Verification items for the finished model (mm, model axes). Face numbers are marked on the shaded views. A direction names the side the tool comes from. Coordinates: 2 decimals unless noted, no trailing zeros. Order: outer loops, then holes, each group sorted by start corner. A loop starts at its lowest first (then second) coordinate and runs counter-clockwise, first axis right, second up. Notation, with made-up numbers: M 78,56 L 104,56 A16 cw 104,63 Z; hole C -11.75,70 d3. An arc over 180 degrees is marked long. Return JSON: item names as keys, results as strings. Group by question number.
Q1. Thickness scan on probe 1 along Y at (x, z) = (-2, 33); probe 2 along Z at (x, y) = (-7.5, 17.5); probe 3 along X at (y, z) = (1, 36.83) (3 decimals). Record the ranges inside material, lowest first.
Q2. Section check B-B, the plane x = 1.25. Enter the section's corners in (y, z).
Q3. Section check A-A, the plane x = 5. Enter the section's corners in (y, z), then the cut area to 3 significant figures.
Q4. Access from +Z, -Z, +X, -X, +Y, -Y to the whole of each face (thin tool, end or side, straight path). Record for the marked faces 1, 2 and 3.
Q5. Section check C-C, the plane z = 36.83. Enter the section's corners in (x, y) (3 decimals).
Q6. Mould release check, pull along Y, two halves, no side actions. Record for the marked faces 4, 5 and 6: pulls with the +Y half, pulls with the -Y half, needs draft (parallel to the pull), parting line crosses it, or undercut.
Q7. Go/stop test with flat-tipped pins: pin 1 Ø1.1 at (x, z) = (6.985, 36.83) entering from +Y; pin 2 Ø2.5 at (y, z) = (-7, 31) entering from -X (3 decimals); pin 3 Ø3 at (y, z) = (-15.5, 29) entering from -X (3 decimals). Record where each tip stops, or that it passes through.
from build123d import *

# Parameters (mm, degrees)
F0_W        = 19.05
F0_H        = 50.8
F1_DEPTH    = 38.1
F2_R        = 5.08
F3_W        = 5.08
F3_H        = 20.32
F4_DEPTH    = 50.8
F5_T        = 2.54
F5_T3_DEPTH = 55.88
F6_R        = 5.07999
F7_R        = 0.635
F8_DEPTH    = 21.59


# Not quite as in the source:
# - a fillet or chamfer is up to 0.001 mm smaller than in the source, because OpenCascade refuses the exact size
# - a shell that OpenCascade refuses in one call is made with other operations: the cavity is built on its own and cut out


with BuildPart() as f1:
    # F0 (on Top) → F1 (new body)
    with BuildSketch(Plane.XY):
        Rectangle(F0_W, F0_H)
    extrude(amount=F1_DEPTH)

    # F2
    f2_edges = [f1.edges().sort_by_distance(p)[0] for p in [
        (0, -25.4, 38.1),
        (0, 25.4, 38.1),
        (-9.525, -25.4, 19.05),
        (-9.525, 0, 38.1),
        (-9.525, 25.4, 19.05),
    ]]
    fillet(f2_edges, radius=F2_R)

    # F3 (on face) → F4 (cut)
    with BuildSketch(Plane.XZ.offset(25.4)):
        with Locations((6.985, 15.24)):
            Rectangle(F3_W, F3_H)
    extrude(amount=-F4_DEPTH, mode=Mode.SUBTRACT)

    # F5: shell of thickness 2.54, made by hand


with BuildPart() as f5_core1:
    # F5_t2: copy of F1
    add(f1.part)

    # the walls: a layer under each face that stays
    f5_faces = [f5_core1.faces().sort_by_distance(p)[0] for p in [
        (2.54, -25.4, 16.51),
        (9.525, 0, 2.54),
        (6.985, 0, 5.08),
        (4.445, 0, 15.24),
        (6.985, 0, 25.4),
        (9.525, 0, 31.75),
        (2.54, -23.9121024484, 36.6121024484),
        (-8.0371024484, -23.9121024484, 16.51),
        (0, 0, 0),
        (2.54, 25.4, 16.51),
        (2.54, 23.9121024484, 36.6121024484),
        (-8.0371024484, -22.86, 35.56),
        (-8.0371024484, 23.9121024484, 16.51),
        (-8.0371024484, 22.86, 35.56),
    ]]
    thicken(f5_faces, amount=-F5_T, mode=Mode.SUBTRACT)

    # F5_s4 → F5_t3 (cut)
    with BuildSketch(Plane.XZ.offset(-27.94)):
        Polygon((4.4704, 5.1054), (4.445, 2.54), (1.905, 2.54), (1.905, 5.08), align=None)
        Polygon((4.4704, 25.3746), (1.905, 25.4), (1.905, 27.94), (4.445, 27.94), align=None)
    extrude(amount=F5_T3_DEPTH, mode=Mode.SUBTRACT)


with BuildPart() as f1_1:
    add(f1.part)

    # what is left inside the walls is the cavity
    f5_cavity = [f5_core1.part.solids().sort_by_distance(p)[0] for p in [
        (-9.4996, 0, 22.86),
    ]]
    add(f5_cavity, mode=Mode.SUBTRACT)

    # F6 (radius 5.08 in the source; OpenCascade refuses exactly that, so slightly less here)
    f6_edges = [f1_1.edges().sort_by_distance(p)[0] for p in [
        (4.445, 0, 5.08),
        (4.445, 0, 25.4),
    ]]
    fillet(f6_edges, radius=F6_R)

    # F7 (on Front) → F8 (cut, symmetric)
    with BuildSketch(Plane.XZ):
        with Locations((6.985, 36.83)):
            Circle(F7_R)
    extrude(amount=F8_DEPTH, both=True, mode=Mode.SUBTRACT)


solid = f1_1.part
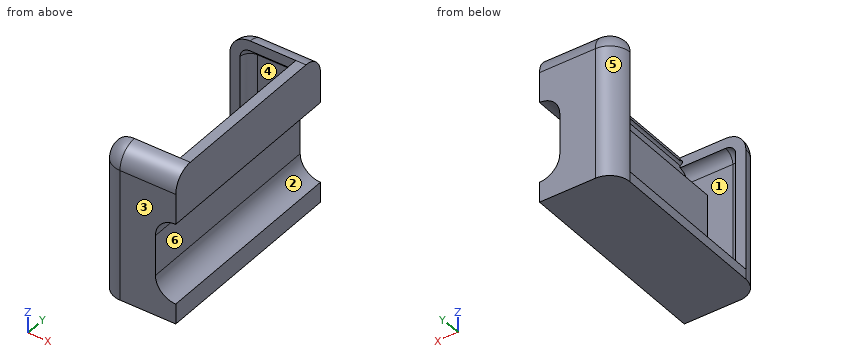
Numbers:
{
 "1": {"probe 1": "y = -25.4 to -22.86, 22.86 to 25.4", "probe 2": "z = 0 to 2.54", "probe 3": "x = 7.62 to 9.525"},
 "2": {"outline": "M -25.4,0 L 25.4,0 L 25.4,33.02 A5.08 ccw 20.32,38.1 L 20.32,35.56 A2.54 cw 22.86,33.02 L 22.86,2.54 L -22.86,2.54 L -22.86,33.02 A2.54 cw -20.32,35.56 L -20.32,38.1 A5.08 ccw -25.4,33.02 Z"},
 "3": {"outline": "M -25.4,0 L 25.4,0 L 25.4,7.85 L -25.4,7.85 Z; M -25.4,22.63 L 25.4,22.63 L 25.4,33.02 A5.08 ccw 20.32,38.1 L 20.32,35.56 A2.54 cw 22.86,33.02 L 22.86,27.94 L -22.86,27.94 L -22.86,33.02 A2.54 cw -20.32,35.56 L -20.32,38.1 A5.08 ccw -25.4,33.02 Z", "area": "725 mm2"},
 "4": {"face 1": "none", "face 2": "+X, +Y, -Y", "face 3": "+Z, -Z, +X, -X, -Y"},
 "5": {"outline": "M -7.805,-20.32 A3.36 ccw -4.445,-23.68 L 9.525,-23.68 L 9.525,23.68 L -4.445,23.68 A3.36 ccw -7.805,20.32 L 6.35,20.32 L 6.35,21.59 L 7.62,21.59 L 7.62,-21.59 L 6.35,-21.59 L 6.35,-20.32 Z"},
 "6": {"face 4": "undercut", "face 5": "pulls with the +Y half", "face 6": "needs draft"},
 "7": {"pin 1": "stops at y = 24.22", "pin 2": "stops at x = 6.985", "pin 3": "stops at x = 1.905"}
}
